```python
from build123d import *

# Parameters (mm, degrees)
SKETCH1_W                  = 444.5
SKETCH1_H                  = 50.8
BOSS_EXTRUDE1_DEPTH        = 0.79375
FILLET1_R                  = 25.4
FILLET2_R                  = 3.175
F_1_0_228_DIAMETER_HOLE1_D = 5.7912


with BuildPart() as part:
    # Sketch1 → Boss-Extrude1 (new body)
    with BuildSketch(Plane(origin=(0, 0, 0), x_dir=(1, 0, 0), z_dir=(0, 1, 0))):
        Rectangle(SKETCH1_W, SKETCH1_H)
    extrude(amount=BOSS_EXTRUDE1_DEPTH)

    # Fillet1
    fillet1_edges = [part.edges().sort_by_distance(p)[0] for p in [
        (222.25, 0.396875, 25.4),
        (-222.25, 0.396875, 25.4),
    ]]
    fillet(fillet1_edges, radius=FILLET1_R)

    # Fillet2
    fillet2_edges = [part.edges().sort_by_distance(p)[0] for p in [
        (-222.25, 0.396875, -25.4),
        (222.25, 0.396875, -25.4),
    ]]
    fillet(fillet2_edges, radius=FILLET2_R)

    # #1 (0.228) Diameter Hole1 (through all)
    with Locations(Plane(origin=(0, 0.79375, 0), x_dir=(1, 0, 0), z_dir=(0, 1, 0))):
        with Locations((166.6875, 12.7), (-166.6875, 12.7)):
            Hole(F_1_0_228_DIAMETER_HOLE1_D / 2)


solid = part.part
```
Geometry check sheet. Reference: the model listing, model coordinates, mm. Round coordinates to 2 decimals unless told otherwise and drop trailing zeros. Order: outer loops, then holes, each group sorted by start corner. A loop starts at its lowest first (then second) coordinate and runs counter-clockwise, first axis right, second up. Notation, with made-up numbers: (24, 27) -> (38, 27) arc R14 cw to (38, 49) -> close; hole circle Ø10 at (66, 44). An arc over 180 degrees is marked (long way). Return JSON: item names as keys, results as strings. Group by question number.
Q1. Section check A-A, the plane z = 21.5. Record the boundary of the cut face in (x, y), plus the area to 3 significant figures.
Q2. Material ranges on probe 1 along X at (y, z) = (0.6, -12.7); probe 2 along X at (y, z) = (0.7, 4.5); probe 3 along X at (y, z) = (0.5, 7), recorded low to high. Write a range as from..to.
Q3. Gauge pin test, flat ends, axial feed: pin 1 (5 mm diameter, centred on x = 166.69, z = -12.7, fed in from +Y); pin 2 (5 mm diameter, centred on x = -155.5, z = 12, fed in from -Y). Record the tip position at first contact, or that the pin passes through.
Numbers:
{
 "1": {"outline": "(-210.37, 0) -> (210.37, 0) -> (210.37, 0.79) -> (-210.37, 0.79) -> close", "area": "334 mm^2"},
 "2": {"probe 1": "-222.25..-169.58, -163.79..163.79, 169.58..222.25", "probe 2": "-221.85..221.85", "probe 3": "-221.27..221.27"},
 "3": {"pin 1": "through", "pin 2": "y = 0"}
}
